For this review, use the dimensioned drawing (mm, ordinates from the lowest corner) and the shaded views. A direction names the side the tool comes from. Coordinates: 2 decimals unless noted, no trailing zeros. Loops run counter-clockwise (first coordinate to the right, second up) from the corner with the lowest first, then second, coordinate; pieces in that order, holes last. Notation, with made-up numbers: M 72,-7.5 L 88,-7.5 A30 cw 88,27.5 Z; hole C 27.25,19.25 d2. An arc over 180 degrees is marked long. One line per item, written item: value.
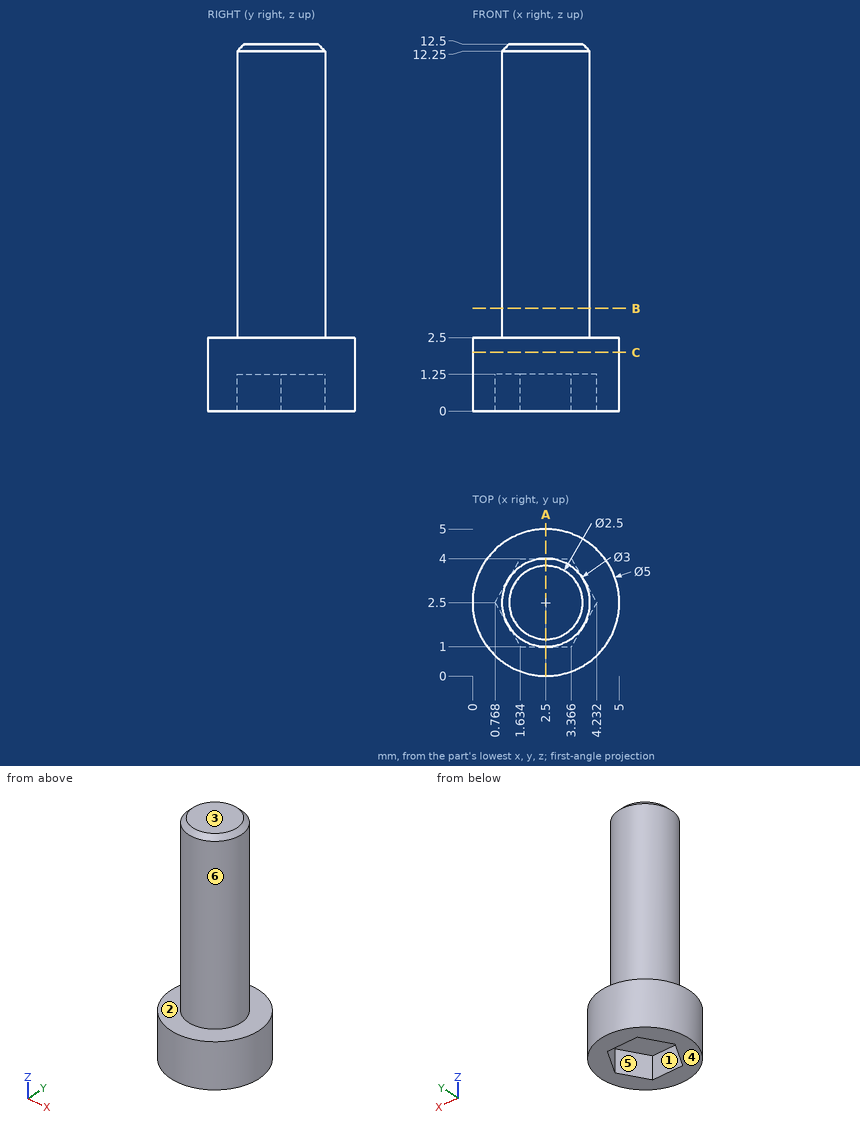
(1) To check wall thickness, follow line 1 along Z through (x, y) = (2.05, 4.7); line 2 along Z through (x, y) = (2.45, 2.65); line 3 along Y through (x, z) = (1.65, 3.25). State the ranges of each line that lie inside material, in increasing order. Write a range as [from, to].
Reply:
line 1: z = [0, 2.5]
line 2: z = [1.25, 12.5]
line 3: y = [1.26, 3.74]
(2) Tool access review of the marked faces 1, 2 and 3: name each direction out of +Z, -Z, +X, -X, +Y, -Y from which nothing blocks a thin tool from reaching the whole face with its end or side.
Reply:
face 1: -Z
face 2: +Z
face 3: +Z, +X, -X, +Y, -Y
(3) Mouldability with a two-part tool opening along X and no side actions: class the marked faces 4, 5 and 6 as released by +X, released by -X, zero draft, split by the parting line, or undercut.
Reply:
face 4: zero draft
face 5: undercut
face 6: split by the parting line
(4) We need section C-C on z = 2. State the section outline as (x, y) points.
Reply:
outline: C 2.5,2.5 d5
(5) We need section A-A on x = 2.5. State the section outline as (y, z) points.
Reply:
outline: M 0,0 L 1,0 L 1,1.25 L 4,1.25 L 4,0 L 5,0 L 5,2.5 L 4,2.5 L 4,12.25 L 3.75,12.5 L 1.25,12.5 L 1,12.25 L 1,2.5 L 0,2.5 Z
(6) We need section B-B on z = 3.5. State the section outline as (x, y) points.
Reply:
outline: C 2.5,2.5 d3
(7) Insertion check: pin 1 (1.5 mm diameter, centred on x = 2, y = 2.5, fed in from -Z); pin 2 (3 mm diameter, centred on x = 0.5, z = 4.5, fed in from -Y). Each pin has a flat end and moves straight along its axis. Give the tip position at first contact, or say it passes through.
Reply:
pin 1: stops at z = 1.25
pin 2: stops at y = 1.09
